Model file for the job. Use its own axes, mm. Face numbers are marked on the shaded views. A direction names the side the tool comes from. Give positions to 0.01 mm unless a question says otherwise; leave off trailing zeros. Order: outer loops, then holes, each group sorted by start corner. A loop starts at its lowest first (then second) coordinate and runs counter-clockwise, first axis right, second up. Notation, with made-up numbers: (5, 5.25) - (34, 5.25) arc R27 cw to (34, 39.25) - close; hole circle Ø11 at (-37.75, -28). An arc over 180 degrees is marked (long way). Return JSON: item names as keys, results as strings. Group by question number.
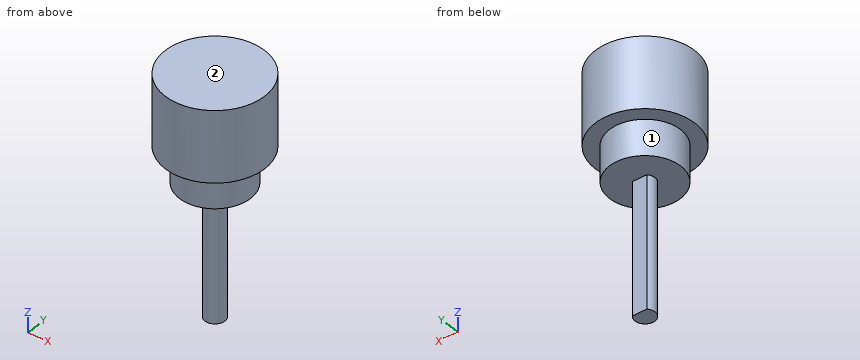
from build123d import *

# Parameters (mm, degrees)
ESQUISSE1_R             = 14
BOSS_EXTRU_1_DEPTH      = 20
BOSS_EXTRU_2_DEPTH      = 47
ESQUISSE3_R             = 18
BOSS_EXTRU_3_DEPTH      = 2
ESQUISSE4_R             = 10
BOSS_EXTRU_4_DEPTH      = 8
BOSS_EXTRU_5_START      = -2
BOSS_EXTRU_5_DEPTH      = 2
ENL_V_START             = -2
ESQUISSE6_R             = 10
ENL_V_MAT_EXTRU_1_DEPTH = 2


with BuildPart() as part:
    # Esquisse1 → Boss.-Extru.1 (new body)
    with BuildSketch(Plane.XY):
        Circle(ESQUISSE1_R)
    extrude(amount=BOSS_EXTRU_1_DEPTH)

    # Esquisse2 → Boss.-Extru.2 (add)
    with BuildSketch(Plane(origin=(0, 0, 0), x_dir=(-1, 0, 0), z_dir=(0, 0, -1))):
        with BuildLine():
            Line((-2.047747609, 1.933319394), (2.047747609, 1.933319394))
            ThreePointArc((2.047747609, 1.933319394), (0, -2.816202079), (-2.047747609, 1.933319394))
        make_face()
    extrude(amount=BOSS_EXTRU_2_DEPTH)

    # Esquisse3 → Boss.-Extru.3 (add)
    with BuildSketch(Plane(origin=(0, 0, 0), x_dir=(-1, 0, 0), z_dir=(0, 0, -1))):
        Circle(ESQUISSE3_R)
    extrude(amount=BOSS_EXTRU_3_DEPTH)

    # Esquisse4 → Boss.-Extru.4 (add)
    with BuildSketch(Plane(origin=(0, 0, -2), x_dir=(-1, 0, 0), z_dir=(0, 0, -1))):
        Circle(ESQUISSE4_R)
    extrude(amount=BOSS_EXTRU_4_DEPTH)

    # Esquisse5 → Boss.-Extru.5 (add)
    with BuildSketch(Plane(origin=(0, 0, -2), x_dir=(-1, 0, 0), z_dir=(0, 0, -1)).offset(BOSS_EXTRU_5_START)):
        with BuildLine():
            Line((50, 18), (0, 18))
            ThreePointArc((0, 18), (12.727922061, 12.727922061), (18, 0))
            ThreePointArc((18, 0), (12.727922061, -12.727922061), (0, -18))
            Line((0, -18), (50, -18))
            ThreePointArc((50, -18), (57.071067812, -15.071067812), (60, -8))
            Line((60, -8), (60, 8))
            ThreePointArc((60, 8), (57.071067812, 15.071067812), (50, 18))
        make_face()
    extrude(amount=BOSS_EXTRU_5_DEPTH)

    # Esquisse6 → Enlèv. mat.-Extru.1 (cut)
    with BuildSketch(Plane(origin=(0, 0, -2), x_dir=(-1, 0, 0), z_dir=(0, 0, -1)).offset(ENL_V_START)):
        Polygon((0, 18), (-22.504594186, 18), (-22.504594186, -18), (62.101973599, -18), (62.101973599, 18), align=None)
        Circle(ESQUISSE6_R, mode=Mode.SUBTRACT)
    extrude(amount=ENL_V_MAT_EXTRU_1_DEPTH, mode=Mode.SUBTRACT)


solid = part.part
(1) Slice it at C-C (z = -32). Give the cut face in (x, y).
(2) Slice it at B-B (y = 0). Give the cut face in (x, z).
(3) 3-axis set-ups, long thin cutter, end or side, ignore diameter. For the marked faces 1 and 2: which of +Z, -Z, +X, -X, +Y, -Y reach the whole face in a straight line?
(4) Slice it at A-A (x = 0). Give the cut face in (y, z).
(5) Drill centre lines: L1, parallel to Z at x = 7, y = -6; L2, parallel to Z at x = -11.75, y = 5.5; L3, parallel to X at y = 0.25, z = -35.5. Where is each one in solid material? Low to high.
(6) Slice it at D-D (x = 5.75). Give the cut face in (y, z).
(7) Drop flat-ended pins along their axis: pin 1 Ø12 at (y, z) = (-10, -28.5) entering from -X; pin 2 Ø10 at (y, z) = (5.5, -5.5) entering from +X; pin 3 Ø1.2 at (x, z) = (1, -29.5) entering from +Y; pin 4 Ø4 at (x, z) = (9.5, 9) entering from -Y. Give the stop position or say it passes through.
Result set:
{
 "1": {"outline": "(-2.05, 1.93) arc R2.82 ccw (long way) to (2.05, 1.93) - close"},
 "2": {"outline": "(-14, 0) - (-10, 0) - (-10, -10) - (-2.82, -10) - (-2.82, -47) - (2.82, -47) - (2.82, -10) - (10, -10) - (10, 0) - (14, 0) - (14, 20) - (-14, 20) - close"},
 "3": {"face 1": "-Z", "face 2": "+Z, +X, -X, +Y, -Y"},
 "4": {"outline": "(-14, 0) - (-10, 0) - (-10, -10) - (-2.82, -10) - (-2.82, -47) - (1.93, -47) - (1.93, -10) - (10, -10) - (10, 0) - (14, 0) - (14, 20) - (-14, 20) - close"},
 "5": {"L1": "z = -10 to 20", "L2": "z = 0 to 20", "L3": "x = -2.81 to 2.81"},
 "6": {"outline": "(-12.76, 0) - (-8.18, 0) - (-8.18, -10) - (8.18, -10) - (8.18, 0) - (12.76, 0) - (12.76, 20) - (-12.76, 20) - close"},
 "7": {"pin 1": "passes through", "pin 2": "stops at x = 9.99", "pin 3": "stops at y = 1.93", "pin 4": "stops at y = -11.82"}
}
